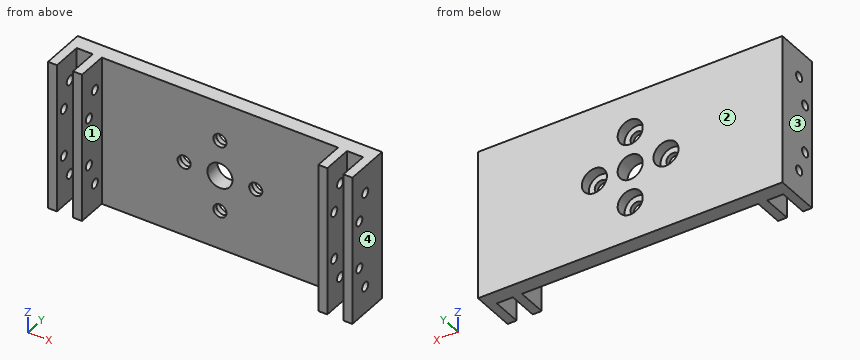
```python
from build123d import *

# Parameters (mm, degrees)
SKETCH4_W           = 102
SKETCH4_H           = 50
SKETCH4_R           = 4.2
SKETCH4_R_2         = 2.2
BOSS_EXTRUDE3_DEPTH = 5
SKETCH16_W          = 3
SKETCH16_H          = 50
BOSS_EXTRUDE4_DEPTH = 10
CUT_EXTRUDE10_REACH = 108.085
SKETCH17_R          = 1.55
CUT_EXTRUDE11_START = -11.4
SKETCH18_R          = 1.55
CUT_EXTRUDE11_DEPTH = 11.4
SKETCH19_R          = 4.2
CUT_EXTRUDE12_DEPTH = 3.5


with BuildPart() as part:
    # Sketch4 → Boss-Extrude3 (new body)
    with BuildSketch(Plane(origin=(0, 0, 0), x_dir=(1, 0, 0), z_dir=(0, 1, 0))):
        Rectangle(SKETCH4_W, SKETCH4_H)
        with Locations(Location((0, 0, 0), (0, 0, 270))):
            Circle(SKETCH4_R, mode=Mode.SUBTRACT)
        with Locations(Location((0, -12, 0), (0, 0, 270))):
            Circle(SKETCH4_R_2, mode=Mode.SUBTRACT)
        with Locations(Location((-12, 0, 0), (0, 0, 270))):
            Circle(SKETCH4_R_2, mode=Mode.SUBTRACT)
        with Locations(Location((0, 12, 0), (0, 0, 270))):
            Circle(SKETCH4_R_2, mode=Mode.SUBTRACT)
        with Locations(Location((12, 0, 0), (0, 0, 270))):
            Circle(SKETCH4_R_2, mode=Mode.SUBTRACT)
    extrude(amount=-BOSS_EXTRUDE3_DEPTH)

    # Sketch16 → Boss-Extrude4 (add)
    with BuildSketch(Plane.XZ.offset(5)):
        with Locations((-41.1, 0)):
            Rectangle(SKETCH16_W, SKETCH16_H)
        with Locations((-49.5, 0)):
            Rectangle(SKETCH16_W, SKETCH16_H)
        with Locations((41.1, 0)):
            Rectangle(SKETCH16_W, SKETCH16_H)
        with Locations((49.5, 0)):
            Rectangle(SKETCH16_W, SKETCH16_H)
    extrude(amount=BOSS_EXTRUDE4_DEPTH)

    # Cut-Extrude10: up to this face of the body (flat: up to its plane)
    cut_extrude10_end = Plane(part.part.faces().sort_by_distance((-39.6, -10, 0))[0])
    # Sketch17 → Cut-Extrude10 (cut, up to the picked face)
    with BuildSketch(Plane.ZY.offset(51), mode=Mode.PRIVATE) as cut_extrude10_sk1:
        with Locations((-16, -8.5)):
            Circle(SKETCH17_R)
    cut_extrude10_tool1 = split(extrude(cut_extrude10_sk1.sketch, amount=-CUT_EXTRUDE10_REACH, mode=Mode.PRIVATE), bisect_by=cut_extrude10_end, keep=Keep.BOTH, mode=Mode.PRIVATE)
    # Sketch17 → Cut-Extrude10 (cut, up to the picked face)
    with BuildSketch(Plane.ZY.offset(51), mode=Mode.PRIVATE) as cut_extrude10_sk2:
        with Locations((-8, -11.5)):
            Circle(SKETCH17_R)
    cut_extrude10_tool2 = split(extrude(cut_extrude10_sk2.sketch, amount=-CUT_EXTRUDE10_REACH, mode=Mode.PRIVATE), bisect_by=cut_extrude10_end, keep=Keep.BOTH, mode=Mode.PRIVATE)
    # Sketch17 → Cut-Extrude10 (cut, up to the picked face)
    with BuildSketch(Plane.ZY.offset(51), mode=Mode.PRIVATE) as cut_extrude10_sk3:
        with Locations((8, -11.5)):
            Circle(SKETCH17_R)
    cut_extrude10_tool3 = split(extrude(cut_extrude10_sk3.sketch, amount=-CUT_EXTRUDE10_REACH, mode=Mode.PRIVATE), bisect_by=cut_extrude10_end, keep=Keep.BOTH, mode=Mode.PRIVATE)
    # Sketch17 → Cut-Extrude10 (cut, up to the picked face)
    with BuildSketch(Plane.ZY.offset(51), mode=Mode.PRIVATE) as cut_extrude10_sk4:
        with Locations((16, -8.5)):
            Circle(SKETCH17_R)
    cut_extrude10_tool4 = split(extrude(cut_extrude10_sk4.sketch, amount=-CUT_EXTRUDE10_REACH, mode=Mode.PRIVATE), bisect_by=cut_extrude10_end, keep=Keep.BOTH, mode=Mode.PRIVATE)
    add(cut_extrude10_tool1.solids().sort_by(Axis((-51, -8.5, -16), (1, 0, 0)))[0], mode=Mode.SUBTRACT)
    add(cut_extrude10_tool2.solids().sort_by(Axis((-51, -11.5, -8), (1, 0, 0)))[0], mode=Mode.SUBTRACT)
    add(cut_extrude10_tool3.solids().sort_by(Axis((-51, -11.5, 8), (1, 0, 0)))[0], mode=Mode.SUBTRACT)
    add(cut_extrude10_tool4.solids().sort_by(Axis((-51, -8.5, 16), (1, 0, 0)))[0], mode=Mode.SUBTRACT)

    # Sketch18 → Cut-Extrude11 (cut)
    with BuildSketch(Plane(origin=(51, 0, 0), x_dir=(0, 0, -1), z_dir=(1, 0, 0)).offset(CUT_EXTRUDE11_START)):
        with Locations(Location((-8, -11.5, 0), (0, 0, 180))):
            Circle(SKETCH18_R)
        with Locations(Location((8, -11.5, 0), (0, 0, 180))):
            Circle(SKETCH18_R)
        with Locations(Location((16, -8.5, 0), (0, 0, 180))):
            Circle(SKETCH18_R)
        with Locations(Location((-16, -8.5, 0), (0, 0, 180))):
            Circle(SKETCH18_R)
    extrude(amount=CUT_EXTRUDE11_DEPTH, mode=Mode.SUBTRACT)

    # Sketch19 → Cut-Extrude12 (cut)
    with BuildSketch(Plane(origin=(0, 0, 0), x_dir=(1, 0, 0), z_dir=(0, 1, 0))):
        with Locations(Location((0, 12, 0), (0, 0, 270))):
            Circle(SKETCH19_R)
        with Locations(Location((12, 0, 0), (0, 0, 270))):
            Circle(SKETCH19_R)
        with Locations(Location((0, -12, 0), (0, 0, 270))):
            Circle(SKETCH19_R)
        with Locations(Location((-12, 0, 0), (0, 0, 270))):
            Circle(SKETCH19_R)
    extrude(amount=-CUT_EXTRUDE12_DEPTH, mode=Mode.SUBTRACT)


solid = part.part
```
Can you work these out from the model? Positions are in its coordinate system, mm. Face numbers are marked on the shaded views. Give positions to 0.01 mm unless a question says otherwise; leave off trailing zeros. Loops run counter-clockwise (first coordinate to the right, second up) from the corner with the lowest first, then second, coordinate; pieces in that order, holes last. Notation, with made-up numbers: M 33,81.5 L 75,81.5 A21 ccw 75,88.5 Z; hole C -25.75,-7.5 d2. An arc over 180 degrees is marked long. One line per question, with ' | ' between items. Start each with the question number.
Q1. If we section it at B-B (z = -12): Please give me the cut outline in (x, y), plus the area to 3 significant figures.
Q2. If we section it at A-A (x = 0): Please give me the cut outline in (y, z).
Q3. If we section it at D-D (y = -1.5): Please give me the cut outline in (x, z), plus the area to 3 significant figures.
Q4. If we section it at C-C (x = -12): Please give me the cut outline in (y, z), plus the area to 3 significant figures.
Q5. If we mould it in two halves opening along X, with no side actions, what happens to the marked faces 1, 2, 3 and 4? For each: +X half, -X half, draft (parallel to the pull), parting line (faces both ways), or undercut.
Q6. If I drill on line 1 (X direction, y = -11.75, z = 5.5); line 2 (Y direction, x = 42, z = 8); line 3 (Z direction, x = 49.9, y = -8.5), over which ranges is the centre line in solid material (lowest first)? Write a range as from..to.
Q7. For pin 1 Ø3 at (y, z) = (-8.5, 16) entering from -X; pin 2 Ø1 at (y, z) = (-12, 9) entering from -X; pin 3 Ø4 at (x, z) = (-11.5, -1.5) entering from +Y; pin 4 Ø7.5 at (x, z) = (0, 12) entering from -Y, each with a flat end and sliding along its axis, tell me the tip position at first contact or that it passes through.
Computed:
1) outline: M -51,-15 L -48,-15 L -48,-5 L -42.6,-5 L -42.6,-15 L -39.6,-15 L -39.6,-5 L -2.2,-5 L -2.2,-3.5 L -4.2,-3.5 L -4.2,0 L -51,0 Z; M 2.2,-5 L 39.6,-5 L 39.6,-15 L 42.6,-15 L 42.6,-5 L 48,-5 L 48,-15 L 51,-15 L 51,0 L 4.2,0 L 4.2,-3.5 L 2.2,-3.5 Z | area: 594 mm²
2) outline: M -5,-25 L 0,-25 L 0,-16.2 L -3.5,-16.2 L -3.5,-14.2 L -5,-14.2 Z; M -5,-9.8 L -3.5,-9.8 L -3.5,-7.8 L 0,-7.8 L 0,-4.2 L -5,-4.2 Z; M -5,4.2 L 0,4.2 L 0,7.8 L -3.5,7.8 L -3.5,9.8 L -5,9.8 Z; M -5,14.2 L -3.5,14.2 L -3.5,16.2 L 0,16.2 L 0,25 L -5,25 Z
3) outline: M -51,-25 L 51,-25 L 51,25 L -51,25 Z; hole C -12,0 d8.4; hole C 0,-12 d8.4; hole C 0,0 d8.4; hole C 0,12 d8.4; hole C 12,0 d8.4 | area: 4,820 mm²
4) outline: M -5,-25 L 0,-25 L 0,-4.2 L -3.5,-4.2 L -3.5,-2.2 L -5,-2.2 Z; M -5,2.2 L -3.5,2.2 L -3.5,4.2 L 0,4.2 L 0,25 L -5,25 Z | area: 214 mm²
5) face 1: undercut | face 2: draft | face 3: -X half | face 4: +X half
6) line 1: x = -51..-48, -42.6..-39.6, 39.6..42.6, 48..51 | line 2: y = -15..-13.05, -9.95..0 | line 3: z = -25..-17.55, -14.45..14.45, 17.55..25
7) pin 1: passes through | pin 2: stops at x = -51 | pin 3: stops at y = -3.5 | pin 4: stops at y = -5
